Model file for the job. Use its own axes, mm. A direction names the side the tool comes from. Round coordinates to 2 decimals unless told otherwise and drop trailing zeros. Order: outer loops, then holes, each group sorted by start corner. A loop starts at its lowest first (then second) coordinate and runs counter-clockwise, first axis right, second up. Notation, with made-up numbers: (73, 82) - (113, 82) arc R19 cw to (113, 108) - close; hole circle Ø10 at (73.5, 60.5). An arc over 180 degrees is marked (long way). Answer as CSV lines item,"result". Start each with the question number.
1. 3-axis set-ups, long thin cutter, end or side, ignore diameter. For faces 4 (the face through (-0.8, -34.88, -1.05)), 5 (the face through (13.955, -20.806, 0.044)): which of +Z, -Z, +X, -X, +Y, -Y reach the whole face in a straight line?
2. Band-saw the part on B-B on z = 2.25. List the corners of the cut face in (x, y) (1 decimal), then the cut area to 3 significant figures.
3. Band-saw the part on A-A on y = 13.5. List the corners of the cut face in (x, z) (3 decimals), then the cut area to 3 significant figures.
4. Band-saw the part on D-D on y = 33. List the corners of the cut face in (x, z) (3 decimals), then the cut area to 3 significant figures.
5. Pin check, flat tips, straight feed: pin 1 Ø2.5 at (x, z) = (0, 0) entering from +Y; pin 2 Ø1.6 at (y, z) = (0, 0) entering from -X; pin 3 Ø1 at (x, z) = (22.5, 0.5) entering from -Y; pin 4 Ø12 at (x, y) = (-12.5, -13) entering from +Z. Stop position of each tip, or through.
6. Pull direction Z, two halves, no side cores. Call faces 1 (the face through (-3, -22, 3.175)), 2 (the face through (-34.88, 0.8, -1.05)), 3 (the face through (13.921, 20.797, 0.044)): released by +Z, released by -Z, zero draft, split by the parting line, or undercut.
7. Wall check: line 1 along Y through (x, z) = (-11, -0.5); line 2 along Y through (x, z) = (7.5, -2); line 3 along X through (y, z) = (-8, 1.75). Give the ranges that are in metal, low to high. Write a range as [from, to].
8. Band-saw the part on C-C on x = 3. List the corners of the cut face in (y, z) (1 decimal).
Autodesk Inventor part; units mm, degrees
ref_plane "Work Plane1" through (0, 38.1, 0) normal (0, 1, 0) x (-1, 0, 0)
ref_plane "YZ Plane" through (0, 0, 0) normal (1, 0, 0) x (0, 1, 0)
ref_plane "XY Plane" through (0, 0, 0) normal (0, 0, 1) x (1, 0, 0)
sketch "Sketch1" plane through (0, 0, 0) normal (0, 0, 1) x (1, 0, 0)
  circle A0 centre (0, 0) radius 38.1
  line L0 (-12.7, 25.4) -> (12.7, 25.4) construction
  line L1 (-12.7, 23.8125) -> (12.7, 23.8125)
  line L2 (12.7, 26.9875) -> (-12.7, 26.9875)
  arc A1 (-12.7, 26.9875) -> (-12.7, 23.8125) centre (-12.7, 25.4) ccw
  arc A2 (12.7, 23.8125) -> (12.7, 26.9875) centre (12.7, 25.4) ccw
  line L3 (0, 38.1) -> (0, -38.1) construction
  line L4 (-38.1, 0) -> (38.1, 0) construction
  line L5 (-12.7, -25.4) -> (12.7, -25.4) construction
  line L6 (-12.7, -23.8125) -> (12.7, -23.8125)
  line L7 (12.7, -26.9875) -> (-12.7, -26.9875)
  arc A3 (-12.7, -23.8125) -> (-12.7, -26.9875) centre (-12.7, -25.4) ccw
  arc A4 (12.7, -26.9875) -> (12.7, -23.8125) centre (12.7, -25.4) ccw
  point P0 (0, 25.4)
  point P1 (0, -25.4)
  dimension "d0" = 76.2
  dimension "d1" = 25.4
  dimension "d2" = 1.5875
  dimension "d3" = 25.4
extrude "Extrusion1" add sketch "Sketch1" along normal mid plane 6.35
sketch "Sketch2" plane through (0, 0, 3.175) normal (0, 0, 1) x (1, 0, 0)
  circle A0 centre (0, 0) radius 38.1 construction
  line L0 (0, 38.1) -> (0, -38.1) construction
  point P0 (-25.4, 0)
  point P1 (25.4, 0)
  dimension "d8" = 25.4
hole "Hole1" at (-25.4, 0, 3.175) at (25.4, 0, 3.175) direction (0, 0, -1) diameter 3.5052 end through all
sketch "Sketch3" plane through (0, 0, 3.175) normal (0, 0, 1) x (1, 0, 0)
  circle A0 centre (25.4, 0) radius 1.7526 construction
  circle A1 centre (-25.4, 0) radius 1.7526 construction
  circle A2 centre (0, 0) radius 38.1 construction
  line L0 (12.7, -26.9875) -> (-12.7, -26.9875) construction
  arc A3 (-12.7, -23.8125) -> (-12.7, -26.9875) centre (-12.7, -25.4) ccw construction
  line L1 (-12.7, -23.8125) -> (12.7, -23.8125) construction
  arc A4 (12.7, -26.9875) -> (12.7, -23.8125) centre (12.7, -25.4) ccw construction
  arc A5 (-12.7, 26.9875) -> (-12.7, 23.8125) centre (-12.7, 25.4) ccw construction
  line L2 (-12.7, 26.9875) -> (12.7, 26.9875) construction
  arc A6 (12.7, 23.8125) -> (12.7, 26.9875) centre (12.7, 25.4) ccw construction
  line L3 (12.7, 23.8125) -> (-12.7, 23.8125) construction
  line L4 (12.7, 30.1625) -> (-12.7, 30.1625)
  arc A7 (-12.7, 30.1625) -> (-12.7, 20.6375) centre (-12.7, 25.4) ccw
  line L5 (-12.7, 20.6375) -> (12.7, 20.6375)
  arc A8 (12.7, 20.6375) -> (12.7, 30.1625) centre (12.7, 25.4) ccw
  circle A9 centre (-25.4, 0) radius 4.9276
  circle A10 centre (25.4, 0) radius 4.9276
  line L6 (12.7, -20.6375) -> (-12.7, -20.6375)
  arc A11 (-12.7, -20.6375) -> (-12.7, -30.1625) centre (-12.7, -25.4) ccw
  line L7 (-12.7, -30.1625) -> (12.7, -30.1625)
  arc A12 (12.7, -30.1625) -> (12.7, -20.6375) centre (12.7, -25.4) ccw
  circle A13 centre (0, 0) radius 33.1606
  arc A14 (-27.6122, 18.3627) -> (-23.4717, 4.5346) centre (-19.8006, 13.1678) ccw
  arc A15 (-23.4717, -4.5346) -> (-27.6122, -18.3627) centre (-19.8006, -13.1678) ccw
  arc A16 (23.4717, 4.5346) -> (27.6122, 18.3627) centre (19.8006, 13.1678) ccw
  arc A17 (27.6122, -18.3627) -> (23.4717, -4.5346) centre (19.8006, -13.1678) ccw
  arc A18 (-27.6122, -18.3627) -> (-15.0909, -21.2812) centre (-19.8006, -13.1678) ccw
  arc A19 (15.0909, -21.2812) -> (27.6122, -18.3627) centre (19.8006, -13.1678) ccw
  arc A20 (-15.0909, 21.2812) -> (-27.6122, 18.3627) centre (-19.8006, 13.1678) ccw
  arc A21 (27.6122, 18.3627) -> (15.0909, 21.2812) centre (19.8006, 13.1678) ccw
  dimension "d16" = 3.175
  dimension "d17" = 3.175
  dimension "d18" = 3.175
  dimension "d19" = 3.175
extrude "Extrusion2" cut sketch "Sketch3" against normal through all contours A21 A16 A10 A17 A19 A12 L6 A11 A18 A15 A9 A14 A20 A7 L5 A8
ref_plane "Work Plane1" through (0, 38.1, 0) normal (0, 1, 0) x (-1, 0, 0)
sketch "Sketch4" plane through (0, 38.1, 0) normal (0, 1, 0) x (-1, 0, 0)
  point P0 (0, 0)
  point P1 (0, 0)
hole "Hole2" at (0, 38.1, 0) direction (0, -1, 0) diameter 2.6416 depth 6.35 tip angle 118
pattern_circular "Circular Pattern1" count 4 over 360 about axis through (0, 0, 0) along (0, 0, 1) of "Hole2"
properties part number "DeploymentBulkhead"
Reply:
1,face 4,"-Y"
1,face 5,"+Z, -Z"
2,outline,"circle Ø76.2 at (0, 0); hole (-27.6, -18.4) arc R9.4 ccw to (-15.1, -21.3) arc R4.8 cw to (-12.7, -20.6) - (12.7, -20.6) arc R4.8 cw to (15.1, -21.3) arc R9.4 ccw to (27.6, -18.4) arc R9.4 ccw to (23.5, -4.5) arc R4.9 cw to (23.5, 4.5) arc R9.4 ccw to (27.6, 18.4) arc R9.4 ccw to (15.1, 21.3) arc R4.8 cw to (12.7, 20.6) - (-12.7, 20.6) arc R4.8 cw to (-15.1, 21.3) arc R9.4 ccw to (-27.6, 18.4) arc R9.4 ccw to (-23.5, 4.5) arc R4.9 cw to (-23.5, -4.5) arc R9.4 ccw to start; hole circle Ø3.5 at (-25.4, 0); hole (-12.7, -27) - (12.7, -27) arc R1.6 ccw to (12.7, -23.8) - (-12.7, -23.8) arc R1.6 ccw to start; hole (-12.7, 23.8) - (12.7, 23.8) arc R1.6 ccw to (12.7, 27) - (-12.7, 27) arc R1.6 ccw to start; hole circle Ø3.5 at (25.4, 0)"
2,area,"2,130 mm2"
3,outline,"(-35.628, -3.175) - (-29.176, -3.175) - (-29.176, 3.175) - (-35.628, 3.175) - close; (29.176, -3.175) - (35.628, -3.175) - (35.628, 3.175) - (29.176, 3.175) - close"
3,area,"81.9 mm2"
4,outline,"(-19.042, -3.175) - (19.042, -3.175) - (19.042, 3.175) - (-19.042, 3.175) - close; hole circle Ø2.642 at (0, 0)"
4,area,"236 mm2"
5,pin 1,"stops at y = 31.71"
5,pin 2,"stops at x = -31.44"
5,pin 3,"stops at y = -31.11"
5,pin 4,"passes through"
6,face 1,"released by +Z"
6,face 2,"undercut"
6,face 3,"zero draft"
7,line 1,"y = [-36.48, -26.99], [-23.81, -20.64], [20.64, 23.81], [26.99, 36.48]"
7,line 2,"y = [-37.35, -26.99], [-23.81, -20.64], [20.64, 23.81], [26.99, 37.35]"
7,line 3,"x = [-37.25, -27.63], [27.63, 37.25]"
8,outline,"(-38, -3.2) - (-27, -3.2) - (-27, 3.2) - (-38, 3.2) - close; (-23.8, -3.2) - (-20.6, -3.2) - (-20.6, 3.2) - (-23.8, 3.2) - close; (20.6, -3.2) - (23.8, -3.2) - (23.8, 3.2) - (20.6, 3.2) - close; (27, -3.2) - (38, -3.2) - (38, 3.2) - (27, 3.2) - close"
